from build123d import *

# Parameters (mm, degrees)
BOSS_EXTRUDE3_DEPTH      = 20
BOSS_EXTRUDE3_DEPTH_BACK = 20
SKETCH4_R                = 8.5
CUT_EXTRUDE1_DEPTH       = 103.622615216
SKETCH5_R                = 1.05
CUT_EXTRUDE2_DEPTH       = 103.622615216
BOSS_EXTRUDE4_START      = -20
SKETCH6_W                = 2
SKETCH6_H                = 42.571067812
BOSS_EXTRUDE4_DEPTH      = 40
CUT_EXTRUDE4_REACH       = 75.867
SKETCH8_R                = 2.125
CUT_EXTRUDE5_DEPTH       = 2
BOSS_EXTRUDE5_DEPTH      = 40
SKETCH10_R               = 1.05
CUT_EXTRUDE6_DEPTH       = 10
CUT_EXTRUDE7_REACH       = 83.049
CUT_EXTRUDE8_DEPTH       = 3


with BuildPart() as part:
    # Sketch3 → Boss-Extrude3 (new, two sides: drawn at the far end of the back side and taken through both)
    with BuildSketch(Plane.XY.offset(-BOSS_EXTRUDE3_DEPTH_BACK)):
        Polygon((-45, 0), (-45, 36.242640687), (-36.171572875, 45.071067812), (36.171572875, 45.071067812), (45, 36.242640687), (45, 0), (45, -2.5), (-45, -2.5), align=None)
        Polygon((-42, 0), (-42, 35), (-34.928932188, 42.071067812), (34.928932188, 42.071067812), (42, 35), (42, 0), (42, -0.5), (-42, -0.5), align=None, mode=Mode.SUBTRACT)
    extrude(amount=BOSS_EXTRUDE3_DEPTH + BOSS_EXTRUDE3_DEPTH_BACK)

    # Sketch4 → Cut-Extrude1 (cut, through all)
    with BuildSketch(Plane.ZY.offset(45)):
        with Locations(Location((0, 9.5, 0), (0, 0, 270))):
            Circle(SKETCH4_R)
    extrude(amount=-CUT_EXTRUDE1_DEPTH, mode=Mode.SUBTRACT)

    # Sketch5 → Cut-Extrude2 (cut, through all)
    with BuildSketch(Plane.ZY.offset(45)):
        with Locations(Location((-8, 32, 0), (0, 0, 270))):
            Circle(SKETCH5_R)
        with Locations(Location((8, 32, 0), (0, 0, 270))):
            Circle(SKETCH5_R)
        with Locations(Location((8, 2, 0), (0, 0, 270))):
            Circle(SKETCH5_R)
        with Locations(Location((-8, 2, 0), (0, 0, 270))):
            Circle(SKETCH5_R)
    extrude(amount=-CUT_EXTRUDE2_DEPTH, mode=Mode.SUBTRACT)

    # Sketch6 → Boss-Extrude4 (add)
    with BuildSketch(Plane.XY.offset(BOSS_EXTRUDE4_START)):
        with Locations((-9, 20.785533906)):
            Rectangle(SKETCH6_W, SKETCH6_H)
        with Locations((9, 20.785533906)):
            Rectangle(SKETCH6_W, SKETCH6_H)
    extrude(amount=BOSS_EXTRUDE4_DEPTH)

    # Cut-Extrude4: up to this face of the body (flat: up to its plane)
    cut_extrude4_end = Plane(part.part.faces().sort_by_distance((10, 20.785533906, 0))[0])
    # Sketch7 → Cut-Extrude4 (cut, up to the picked face)
    with BuildSketch(Plane.ZY.offset(10), mode=Mode.PRIVATE) as cut_extrude4_sk1:
        Polygon((-20, 26), (-20, 6), (-11, 15), (-11, 17), align=None)
    cut_extrude4_tool1 = split(extrude(cut_extrude4_sk1.sketch, amount=-CUT_EXTRUDE4_REACH, mode=Mode.PRIVATE), bisect_by=cut_extrude4_end, keep=Keep.BOTH, mode=Mode.PRIVATE)
    cut_extrude4 = cut_extrude4_tool1.solids().sort_by(Axis((-10, 16, -16.727273), (1, 0, 0)))[0]
    add(cut_extrude4, mode=Mode.SUBTRACT)

    # Mirror1: Cut-Extrude4 across plane
    add(cut_extrude4.mirror(Plane.XY), mode=Mode.SUBTRACT)

    # Sketch8 → Cut-Extrude5 (cut)
    with BuildSketch(Plane.ZY.offset(45)):
        with Locations(Location((-8, 32, 0), (0, 0, 270))):
            Circle(SKETCH8_R)
        with Locations(Location((8, 32, 0), (0, 0, 270))):
            Circle(SKETCH8_R)
        with Locations(Location((8, 2, 0), (0, 0, 270))):
            Circle(SKETCH8_R)
        with Locations(Location((-8, 2, 0), (0, 0, 270))):
            Circle(SKETCH8_R)
    cut_extrude5 = extrude(amount=-CUT_EXTRUDE5_DEPTH, mode=Mode.SUBTRACT)

    # Mirror2: Cut-Extrude5 across plane
    add(cut_extrude5.mirror(Plane(origin=(0, 0, 0), x_dir=(0, 0, 1), z_dir=(1, 0, 0))), mode=Mode.SUBTRACT)

    # Sketch9 → Boss-Extrude5 (add)
    with BuildSketch(Plane.XY.offset(20)):
        Polygon((17, 55.071067812), (16, 56.071067812), (15, 56.071067812), (14, 55.071067812), (14, 45.071067812), (17, 45.071067812), align=None)
    boss_extrude5 = extrude(amount=-BOSS_EXTRUDE5_DEPTH)

    # Mirror3: Boss-Extrude5 across plane
    add(boss_extrude5.mirror(Plane(origin=(0, 0, 0), x_dir=(0, 0, 1), z_dir=(1, 0, 0))))

    # Sketch10 → Cut-Extrude6 (cut)
    with BuildSketch(Plane(origin=(0, 56.071067812, 0), x_dir=(1, 0, 0), z_dir=(0, 1, 0))):
        with Locations(Location((-15.5, 15.5, 0), (0, 0, 180))):
            Circle(SKETCH10_R)
        with Locations(Location((15.5, 15.5, 0), (0, 0, 180))):
            Circle(SKETCH10_R)
        with Locations(Location((15.5, -15.5, 0), (0, 0, 180))):
            Circle(SKETCH10_R)
        with Locations(Location((-15.5, -15.5, 0), (0, 0, 180))):
            Circle(SKETCH10_R)
    extrude(amount=-CUT_EXTRUDE6_DEPTH, mode=Mode.SUBTRACT)

    # Cut-Extrude7: up to this face of the body (flat: up to its plane)
    cut_extrude7_end = Plane(part.part.faces().sort_by_distance((10, 21.415191548, 0))[0])
    # Sketch11 → Cut-Extrude7 (cut, up to the picked face)
    with BuildSketch(Plane.ZY.offset(10), mode=Mode.PRIVATE) as cut_extrude7_sk1:
        with BuildLine():
            Line((-7.5, 40.071067812), (7.5, 40.071067812))
            ThreePointArc((7.5, 40.071067812), (8.55, 39.021067812), (7.5, 37.971067812))
            Line((7.5, 37.971067812), (-7.5, 37.971067812))
            ThreePointArc((-7.5, 37.971067812), (-8.55, 39.021067812), (-7.5, 40.071067812))
        make_face()
    cut_extrude7_tool1 = split(extrude(cut_extrude7_sk1.sketch, amount=-CUT_EXTRUDE7_REACH, mode=Mode.PRIVATE), bisect_by=cut_extrude7_end, keep=Keep.BOTH, mode=Mode.PRIVATE)
    # Sketch11 → Cut-Extrude7 (cut, up to the picked face)
    with BuildSketch(Plane.ZY.offset(10), mode=Mode.PRIVATE) as cut_extrude7_sk2:
        with BuildLine():
            Line((-7.5, 3.5), (7.5, 3.5))
            ThreePointArc((7.5, 3.5), (8.5, 2.5), (7.5, 1.5))
            Line((7.5, 1.5), (-7.5, 1.5))
            ThreePointArc((-7.5, 1.5), (-8.5, 2.5), (-7.5, 3.5))
        make_face()
    cut_extrude7_tool2 = split(extrude(cut_extrude7_sk2.sketch, amount=-CUT_EXTRUDE7_REACH, mode=Mode.PRIVATE), bisect_by=cut_extrude7_end, keep=Keep.BOTH, mode=Mode.PRIVATE)
    add(cut_extrude7_tool1.solids().sort_by(Axis((-10, 39.021068, 0), (1, 0, 0)))[0], mode=Mode.SUBTRACT)
    add(cut_extrude7_tool2.solids().sort_by(Axis((-10, 2.5, 0), (1, 0, 0)))[0], mode=Mode.SUBTRACT)

    # Sketch12 → Cut-Extrude8 (cut)
    with BuildSketch(Plane(origin=(0, 45.071067812, 0), x_dir=(1, 0, 0), z_dir=(0, 1, 0))):
        Polygon((-7, 12), (-7, -12), (-1, -18), (1, -18), (7, -12), (7, 12), (1, 18), (-1, 18), align=None)
    extrude(amount=-CUT_EXTRUDE8_DEPTH, mode=Mode.SUBTRACT)


solid = part.part
The model under review builds one solid part; all positions refer to its coordinate system, in mm. A direction names the side the tool comes from. Give positions to 0.01 mm unless a question says otherwise; leave off trailing zeros. Write each loop counter-clockwise with the first axis right and the second up, starting at its lowest first coordinate (ties: lowest second). Pieces come first, ordered by that corner, then holes.
1. Tool access review of faces 5 (the flat face through (0, 44, 18)), 6 (the cylindrical face through (-44.01, 3.69, 6.71)), 7 (the flat face through (17, 50, 0)): name each direction out of +Z, -Z, +X, -X, +Y, -Y from which nothing blocks a thin tool from reaching the whole face with its end or side.
2. Wall thickness on L1, parallel to X at y = 13.5, z = 12; L2, parallel to Z at x = -15.5, y = 51.5; L3, parallel to Z at x = 44.25, y = 32 (3 decimals): over which ranges is each line inside the solid? List them lowest first.
3. Add section A-A, the plane x = 21. Write out the cut boundary in (y, z), plus the area to 3 significant figures.
4. Draft analysis for pull direction Y (two halves, no side actions). For faces 1 (the cylindrical face through (43.479, 16.245, -5.172)), 2 (the flat face through (26, 45.071, 0)), 3 (the flat face through (9, 16, 11)), 4 (the flat face through (-4, 44, -15)), state which applies: +Y half, -Y half, draft (parallel to the pull), parting line (faces both ways), or undercut.
5. For P1, Ø6, axis at y = 4.5, z = 2.5, coming from the -X side; P2, Ø4, axis at y = 2, z = 8, coming from the -X side; P3, Ø4, axis at x = 7.5, z = -7.5, coming from the +Y side; P4, Ø6, axis at y = 44, z = 9.5, coming from the -X side, all flat-tipped, find the tip position at first contact; note any pin that passes through.
6. Add section D-D, the plane z = 0. Count the separate pieces of the cut face and the enclosed holes in it, plus the area to 3 significant figures.
7. Add section B-B, the plane y = 21.5. Write out the cut boundary in (x, z).
8. Add section C-C, the plane y = 51. Write out the cut boundary in (x, z).
Worked answers:
1. face 5: +Y
1. face 6: -X
1. face 7: +Z, -Z, +X, +Y
2. L1: x = -45 to -42, -10 to -8, 8 to 10, 42 to 45
2. L2: z = -20 to -16.55, -14.45 to 14.45, 16.55 to 20
2. L3: z = -20 to -10.125, -5.875 to 5.875, 10.125 to 20
3. outline: (-2.5, -20) - (-0.5, -20) - (-0.5, 20) - (-2.5, 20) - close; (42.07, -20) - (45.07, -20) - (45.07, 20) - (42.07, 20) - close
3. area: 200 mm2
4. face 1: undercut
4. face 2: +Y half
4. face 3: undercut
4. face 4: draft
5. P1: stops at x = -45
5. P2: stops at x = -43
5. P3: stops at y = 45.07
5. P4: stops at x = -40.24
6. separate pieces: 5
6. enclosed holes: 0
6. area: 751 mm2
7. outline: (-45, -20) - (-42, -20) - (-42, 20) - (-45, 20) - close; (-10, -15.5) - (-8, -15.5) - (-8, 15.5) - (-10, 15.5) - close; (8, -15.5) - (10, -15.5) - (10, 15.5) - (8, 15.5) - close; (42, -20) - (45, -20) - (45, 20) - (42, 20) - close
8. outline: (-17, -20) - (-14, -20) - (-14, 20) - (-17, 20) - close; (14, -20) - (17, -20) - (17, 20) - (14, 20) - close; hole circle Ø2.1 at (-15.5, -15.5); hole circle Ø2.1 at (-15.5, 15.5); hole circle Ø2.1 at (15.5, -15.5); hole circle Ø2.1 at (15.5, 15.5)
